Autodesk Inventor part; units mm, degrees
ref_plane "YZ Plane" through (0, 0, 0) normal (1, 0, 0) x (0, 1, 0)
ref_plane "XZ Plane" through (0, 0, 0) normal (0, 1, 0) x (-1, 0, 0)
ref_plane "XY Plane" through (0, 0, 0) normal (0, 0, 1) x (1, 0, 0)
sketch "Sketch1" plane through (0, 0, 0) normal (0, 1, 0) x (-1, 0, 0)
  line L0 (0, 0) -> (80, 0)
  line L1 (80, 0) -> (80, -150)
  line L2 (80, -150) -> (0, -150)
  line L3 (0, -150) -> (0, 0)
  dimension "d0" = 80
  dimension "d1" = 150
extrude "Extrusion1" add sketch "Sketch1" along normal blind 140
sketch "Sketch2" plane through (0, 0, 0) normal (1, 0, 0) x (0, 0, -1)
  line L0 (150, 140) -> (0, 140)
  line L1 (15.8986, 80) -> (79.9832, 29)
  line L2 (79.9832, 29) -> (79.9832, 14)
  line L3 (79.9832, 14) -> (142.2187, 14)
  line L4 (142.2187, 14) -> (142.2187, 44)
  line L5 (142.2187, 44) -> (150, 44)
  line L6 (150, 0) -> (150, 140)
  line L7 (150, 44) -> (150, 140)
  line L8 (150, 140) -> (61.0962, 140)
  line L9 (15.8986, 100) -> (15.8986, 80)
  line L10 (0, 0) -> (150, 0)
  line L11 (61.0962, 140) -> (15.8986, 140)
  line L12 (15.8986, 100) -> (15.8986, 140)
  point P0 (146.1093, 44)
  point P1 (111.101, 14)
  dimension "d7" = 15
  dimension "d8" = 30
  dimension "d9" = 14
extrude "Extrusion2" cut sketch "Sketch2" against normal blind 140
sketch "Sketch6" plane through (0, 14, -79.9832) normal (0, 1, 0) x (1, 0, 0)
  line L0 (0, 62.2355) -> (-80, 62.2355)
  line L1 (0, 0) -> (-80, 0)
  line L2 (-80, 62.2355) -> (-75.5003, 62.2355)
  line L3 (-75.5003, 62.2355) -> (-75.5003, 0)
  line L4 (-75.5003, 0) -> (-80, 0)
  line L5 (-80, 0) -> (-80, 62.2355)
  point P0 (0, -79.9832)
extrude "Extrusion6" add sketch "Sketch6" along normal blind 15
properties part number "Left"
Model file for the job. Use its own axes, mm. A direction names the side the tool comes from. Give positions to 0.01 mm unless a question says otherwise; leave off trailing zeros. Order: outer loops, then holes, each group sorted by start corner. A loop starts at its lowest first (then second) coordinate and runs counter-clockwise, first axis right, second up. Notation, with made-up numbers: (31.5, -25) - (38.5, -25) arc R19 ccw to (38.5, -3) - close; hole circle Ø3 at (88, 9). An arc over 180 degrees is marked (long way). One line per item, written item: value.
Item 1: Tool access for faces 1 (the flat face through (-75.5, 21, -112)), 2 (the flat face through (-78, 29, -112)), 3 (the flat face through (-39, 44, -146)): list every direction of +Z, -Z, +X, -X, +Y, -Y with a clear straight run to the whole face (end or side of a thin tool).
Response values:
face 1: +X, +Y
face 2: +X, -X, +Y
face 3: -Z, +X, -X, +Y
Item 2: Slice it at A-A (x = -61.5). List the corners of the cut face in (y, z).
Response values:
outline: (0, -150) - (44, -150) - (44, -142.22) - (14, -142.22) - (14, -79.98) - (29, -79.98) - (80, -15.9) - (140, -15.9) - (140, 0) - (0, 0) - close
Item 3: Slice it at C-C (y = 130). List the corners of the cut face in (x, z), then the cut area to 3 significant figures.
Response values:
outline: (-80, -15.9) - (0, -15.9) - (0, 0) - (-80, 0) - close
area: 1,270 mm2
Item 4: Wall check: line 1 (Z direction, x = -29.5, y = 27); line 2 (Z direction, x = -9, y = 104); line 3 (Y direction, x = -48, z = -120). Give the ranges that are in metal, low to high.
Response values:
line 1: -150 to -142.22, -79.98 to 0
line 2: -15.9 to 0
line 3: 0 to 14
Item 5: Two-plate mould, pull along Z, no slides. Class faces 4 (the flat face through (-39.44, 54.86, -47.49)), 5 (the flat face through (-39, 140, -8)), 6 (the flat face through (-39, 110, -15.899)): released by +Z, released by -Z, zero draft, split by the parting line, or undercut.
Response values:
face 4: undercut
face 5: zero draft
face 6: released by -Z
Item 6: Slice it at B-B (z = -129.5). List the corners of the cut face in (x, y).
Response values:
outline: (-80, 0) - (0, 0) - (0, 14) - (-75.5, 14) - (-75.5, 29) - (-80, 29) - close
Item 7: Pin check, flat tips, straight feed: pin 1 Ø18.5 at (x, z) = (-47.5, -97) entering from +Y; pin 2 Ø12 at (y, z) = (24.5, -100) entering from +X; pin 3 Ø2 at (x, z) = (-77, -120) entering from +Y. Stop position of each tip, or through.
Response values:
pin 1: y = 14
pin 2: x = -75.5
pin 3: y = 29
Item 8: Slice it at D-D (z = -63.5). List the corners of the cut face in (x, y), then the cut area to 3 significant figures.
Response values:
outline: (-80, 0) - (0, 0) - (0, 42.12) - (-80, 42.12) - close
area: 3,370 mm2
